The figure shows three views and two pictorial views of one solid part (mm, origin at its lowest corner). Answer the questions. Give positions to 0.01 mm unless a question says otherwise; leave off trailing zeros. Order: outer loops, then holes, each group sorted by start corner. A loop starts at its lowest first (then second) coordinate and runs counter-clockwise, first axis right, second up. Notation, with made-up numbers: (20.25, 34) - (60.25, 34) arc R27 ccw to (60.25, 67) - close; hole circle Ø4 at (34, 86). An arc over 180 degrees is marked (long way). Answer as CSV lines item,"result". Start each with the question number.
1. Section C-C on y = 3.25 is taken. Give the vertices of the cut face in (x, z).
2. Section B-B on x = 4 is taken. Give the vertices of the cut face in (y, z), and give its area (3 significant figures).
3. Determine the mould class of the marked faces 1, 2, 3 and 4 for opening direction Y: +Y half, -Y half, draft (parallel to the pull), parting line (faces both ways), or undercut.
4. Consider line 1 along Y through (x, z) = (4, 0.5); line 2 along Y through (x, z) = (2.75, 0.2); line 3 along X through (y, z) = (5.75, 1.7) (1 decimal). Determine where each line is inside the solid, lowest interval first. Write a range as [from, to].
5. Section A-A on z = 1.7 is taken. Give the vertices of the cut face in (x, y), and give its area (3 significant figures).
6. Section D-D on y = 10.25 is taken. Give the vertices of the cut face in (x, z).
7. Flat-ended cylindrical pins translate along their axes: pin 1 (1 mm diameter, centred on y = 9, z = 1.5, fed in from +X); pin 2 (1 mm diameter, centred on x = 6.5, z = 1, fed in from +Y) (1 decimal); pin 3 (1 mm diameter, centred on y = 7, z = 0.5, fed in from -X). Find the tip coordinate at first contact, or state that the pin passes through.
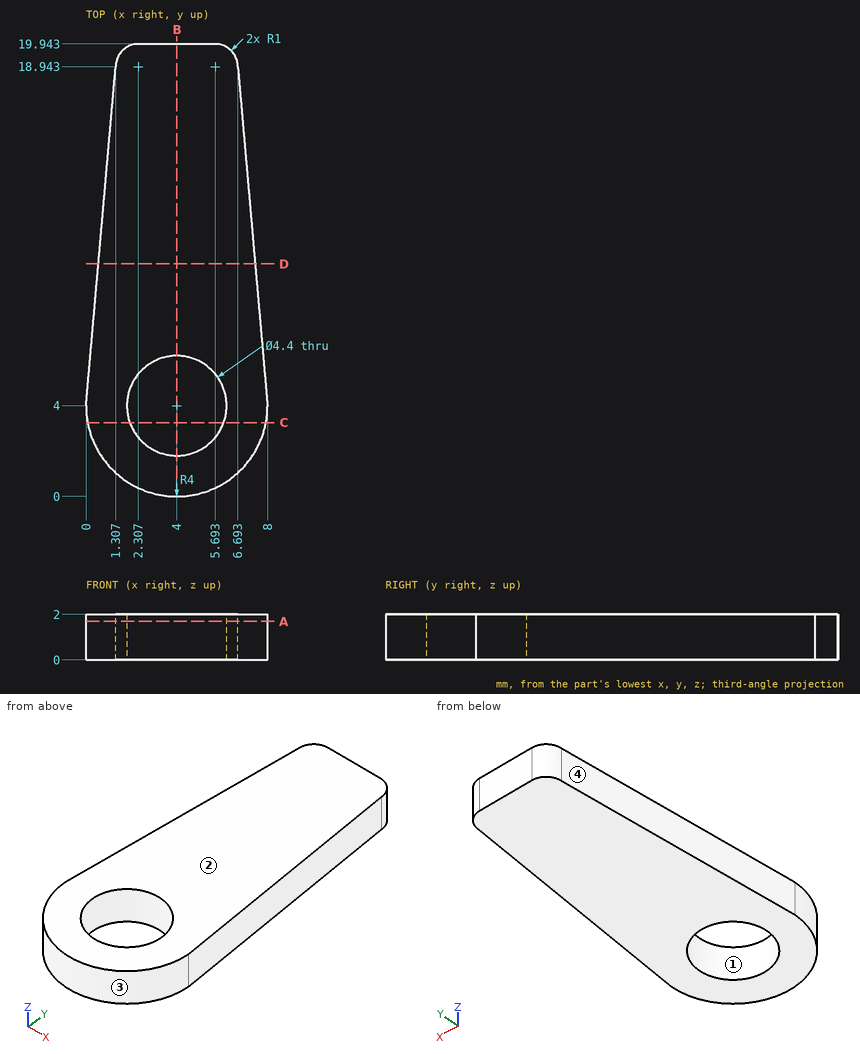
Checks:
1,outline,"(0.07, 0) - (1.93, 0) - (1.93, 2) - (0.07, 2) - close; (6.07, 0) - (7.93, 0) - (7.93, 2) - (6.07, 2) - close"
2,outline,"(0, 0) - (1.8, 0) - (1.8, 2) - (0, 2) - close; (6.2, 0) - (19.94, 0) - (19.94, 2) - (6.2, 2) - close"
2,area,"31.1 mm²"
3,face 1,"undercut"
3,face 2,"draft"
3,face 3,"-Y half"
3,face 4,"+Y half"
4,line 1,"y = [0, 1.8], [6.2, 19.94]"
4,line 2,"y = [0.2, 2.19], [5.81, 19.94]"
4,line 3,"x = [0.2, 2.7], [5.3, 7.8]"
5,outline,"(0, 4) arc R4 ccw to (8, 4) - (6.69, 18.94) arc R1 ccw to (5.69, 19.94) - (2.31, 19.94) arc R1 ccw to (1.31, 18.94) - close; hole circle Ø4.4 at (4, 4)"
5,area,"115 mm²"
6,outline,"(0.55, 0) - (7.45, 0) - (7.45, 2) - (0.55, 2) - close"
7,pin 1,"stops at x = 7.61"
7,pin 2,"stops at y = 19.9"
7,pin 3,"stops at x = 0.22"
